from build123d import *

# Parameters (mm, degrees)
BOSS_EXTRUDE1_DEPTH     = 8
FILLET1_R               = 3
CUT_EXTRUDE1_DEPTH      = 90.03548582
CUT_EXTRUDE2_DEPTH      = 90.03548582
CUT_EXTRUDE2_DEPTH_BACK = 90.03548582
FILLET2_R               = 3
SKETCH4_R               = 1.5
CUT_EXTRUDE3_DEPTH      = 90.03548582
SKETCH5_R               = 2.5
CUT_EXTRUDE4_DEPTH      = 3
SKETCH7_W               = 100
SKETCH7_H               = 30
BOSS_EXTRUDE2_DEPTH     = 8
SKETCH8_W               = 15
SKETCH8_H               = 20
BOSS_EXTRUDE3_DEPTH     = 23
SKETCH9_R               = 2.5
CUT_EXTRUDE5_DEPTH      = 20
FILLET3_R               = 7.5
FILLET4_R               = 3
FILLET5_R               = 3
CUT_EXTRUDE6_DEPTH      = 142.723882577
CUT_EXTRUDE7_DEPTH      = 5
SKETCH12_W              = 15
SKETCH12_H              = 6
CUT_EXTRUDE8_DEPTH      = 5
SKETCH13_W              = 15
SKETCH13_H              = 6
CUT_EXTRUDE9_DEPTH      = 5
FILLET6_R               = 5


with BuildPart() as part:
    # Sketch1 → Boss-Extrude1 (new body)
    with BuildSketch(Plane(origin=(0, 0, 0), x_dir=(1, 0, 0), z_dir=(0, 1, 0))):
        Polygon((-10, 25), (0, 75), (10, 25), (25, 25), (25, 10), (75, 0), (25, -10), (25, -25), (10, -25), (0, -75), (-10, -25), (-25, -25), (-25, -10), (-75, 0), (-25, 10), (-25, 25), align=None)
    extrude(amount=BOSS_EXTRUDE1_DEPTH)

    # Fillet1
    fillet1_edges = [part.edges().sort_by_distance(p)[0] for p in [
        (0, 4, -75),
        (75, 4, 0),
        (0, 4, 75),
        (-75, 4, 0),
    ]]
    fillet(fillet1_edges, radius=FILLET1_R)

    # Sketch2 → Cut-Extrude1 (cut, symmetric)
    with BuildSketch(Plane(origin=(0, 0, 0), x_dir=(0, 0, -1), z_dir=(1, 0, 0))):
        Polygon((25, 8), (62.702941459, 2), (62.702941459, 8), align=None)
    cut_extrude1 = extrude(amount=CUT_EXTRUDE1_DEPTH, both=True, mode=Mode.SUBTRACT)

    # Mirror2: Cut-Extrude1 across plane
    add(cut_extrude1.mirror(Plane.XY), mode=Mode.SUBTRACT)

    # Sketch3 → Cut-Extrude2 (cut, two sides: drawn at the far end of the back side and taken through both)
    with BuildSketch(Plane.XY.offset(-CUT_EXTRUDE2_DEPTH_BACK)):
        Polygon((-25, 8), (-62.702941459, 2), (-62.702941459, 8), align=None)
    extrude(amount=CUT_EXTRUDE2_DEPTH + CUT_EXTRUDE2_DEPTH_BACK, mode=Mode.SUBTRACT)

    # Fillet2
    fillet2_edges = [part.edges().sort_by_distance(p)[0] for p in [
        (-10, 4, -25),
        (10, 4, -25),
        (25, 4, -25),
        (25, 4, 25),
        (10, 4, 25),
        (-10, 4, 25),
        (-25, 4, 25),
        (-25, 4, 10),
        (-25, 4, -10),
        (-25, 4, -25),
    ]]
    fillet(fillet2_edges, radius=FILLET2_R)

    # Sketch4 → Cut-Extrude3 (cut, through all)
    with BuildSketch(Plane(origin=(0, 8, 0), x_dir=(1, 0, 0), z_dir=(0, 1, 0))):
        with Locations(Location((-15.5, 15.5, 0), (0, 0, 270))):
            Circle(SKETCH4_R)
        with Locations(Location((15.5, 15.5, 0), (0, 0, 270))):
            Circle(SKETCH4_R)
        with Locations(Location((15.5, -15.5, 0), (0, 0, 270))):
            Circle(SKETCH4_R)
        with Locations(Location((-15.5, -15.5, 0), (0, 0, 270))):
            Circle(SKETCH4_R)
    extrude(amount=-CUT_EXTRUDE3_DEPTH, mode=Mode.SUBTRACT)

    # Sketch5 → Cut-Extrude4 (cut)
    with BuildSketch(Plane.XZ):
        with Locations(Location((15.5, -15.5, 0), (0, 0, 270))):
            Circle(SKETCH5_R)
        with Locations(Location((-15.5, -15.5, 0), (0, 0, 270))):
            Circle(SKETCH5_R)
        with Locations(Location((-15.5, 15.5, 0), (0, 0, 270))):
            Circle(SKETCH5_R)
        with Locations(Location((15.5, 15.5, 0), (0, 0, 270))):
            Circle(SKETCH5_R)
    extrude(amount=-CUT_EXTRUDE4_DEPTH, mode=Mode.SUBTRACT)

    # Sketch7 → Boss-Extrude2 (add)
    with BuildSketch(Plane(origin=(0, 8, 0), x_dir=(1, 0, 0), z_dir=(0, 1, 0))):
        with Locations((75, 0)):
            Rectangle(SKETCH7_W, SKETCH7_H)
    extrude(amount=-BOSS_EXTRUDE2_DEPTH)

    # Sketch8 → Boss-Extrude3 (add)
    with BuildSketch(Plane(origin=(0, 8, 0), x_dir=(1, 0, 0), z_dir=(0, 1, 0))):
        with Locations((117.5, 0)):
            Rectangle(SKETCH8_W, SKETCH8_H)
    extrude(amount=BOSS_EXTRUDE3_DEPTH)

    # Sketch9 → Cut-Extrude5 (cut)
    with BuildSketch(Plane.XY.offset(10)):
        with Locations((117.5, 25)):
            Circle(SKETCH9_R)
    extrude(amount=-CUT_EXTRUDE5_DEPTH, mode=Mode.SUBTRACT)

    # Fillet3
    fillet3_edges = [part.edges().sort_by_distance(p)[0] for p in [
        (110, 31, 0),
        (125, 31, 0),
    ]]
    fillet(fillet3_edges, radius=FILLET3_R - 0.0001)  # a hair under: the kernel refuses the full size

    # Fillet4
    fillet4_edges = [part.edges().sort_by_distance(p)[0] for p in [
        (117.5, 8, -10),
        (117.5, 8, 10),
    ]]
    fillet(fillet4_edges, radius=FILLET4_R)

    # Fillet5
    fillet5_edges = [part.edges().sort_by_distance(p)[0] for p in [
        (125, 4, 15),
        (125, 4, -15),
    ]]
    fillet(fillet5_edges, radius=FILLET5_R)

    # Sketch10 → Cut-Extrude6 (cut, through all)
    with BuildSketch(Plane(origin=(0, 8, 0), x_dir=(1, 0, 0), z_dir=(0, 1, 0))):
        Polygon((30, -8), (91.024338464, -8), (30, 5.94842022), align=None)
        Polygon((38.975661536, 8), (100, 8), (100, -5.94842022), align=None)
        Polygon((9.085786438, 10.5), (0, 1.414213562), (-9.085786438, 10.5), align=None)
        Polygon((10.5, -9.085786438), (1.414213562, 0), (10.5, 9.085786438), align=None)
        Polygon((-9.085786438, -10.5), (0, -1.414213562), (9.085786438, -10.5), align=None)
        Polygon((-10.5, 9.085786438), (-1.414213562, 0), (-10.5, -9.085786438), align=None)
    extrude(amount=-CUT_EXTRUDE6_DEPTH, mode=Mode.SUBTRACT)

    # Sketch11 → Cut-Extrude7 (cut)
    with BuildSketch(Plane.XY.offset(10)):
        with BuildLine():
            Line((109, 25), (109, 32))
            Line((109, 32), (126, 32))
            Line((126, 32), (126, 25))
            ThreePointArc((126, 25), (117.5, 16.5), (109, 25))
        make_face()
    cut_extrude7 = extrude(amount=-CUT_EXTRUDE7_DEPTH, mode=Mode.SUBTRACT)

    # Mirror4: Cut-Extrude7 across plane
    add(cut_extrude7.mirror(Plane.XY), mode=Mode.SUBTRACT)

    # Sketch12 → Cut-Extrude8 (cut)
    with BuildSketch(Plane.XY.offset(10)):
        with Locations((117.5, 18)):
            Rectangle(SKETCH12_W, SKETCH12_H)
    extrude(amount=-CUT_EXTRUDE8_DEPTH, mode=Mode.SUBTRACT)

    # Sketch13 → Cut-Extrude9 (cut)
    with BuildSketch(Plane(origin=(0, 0, -10), x_dir=(-1, 0, 0), z_dir=(0, 0, -1))):
        with Locations((-117.5, 18)):
            Rectangle(SKETCH13_W, SKETCH13_H)
    extrude(amount=-CUT_EXTRUDE9_DEPTH, mode=Mode.SUBTRACT)

    # Fillet6
    fillet6_edges = [part.edges().sort_by_distance(p)[0] for p in [
        (125, 15, -7.5),
        (110, 15, -7.5),
        (110, 15, 7.5),
        (125, 15, 7.5),
    ]]
    fillet(fillet6_edges, radius=FILLET6_R)


solid = part.part
Read the model definition and answer for the solid it produces. Units are mm, in the model's axes. A direction names the side the tool comes from. Round coordinates to 2 decimals unless told otherwise and drop trailing zeros. Write each loop counter-clockwise with the first axis right and the second up, starting at its lowest first coordinate (ties: lowest second). Pieces come first, ordered by that corner, then holes.
Q1. Find section A-A on x = 42. Determine the outline of the cut face in (y, z).
Values:
outline: (0, -15) - (8, -15) - (8, -8) - (0, -8) - close; (0, -7.31) - (8, -7.31) - (8, -3.21) - (0, -3.21) - close; (0, 8) - (8, 8) - (8, 15) - (0, 15) - close
Q2. A tool of negligible diameter and unlimited length cuts with its end or side. For faces 5 (the face through (0, 4, 10.5)), 6 (the face through (-17, 3, -17)), 7 (the face through (125, 9, 0)), from which of +Z, -Z, +X, -X, +Y, -Y can it reach the whole face along a straight path? Write none if from no direction.
Values:
face 5: +Y, -Y
face 6: -Y
face 7: +Z, -Z, +X, +Y, -Y
Q3. Straight lines are drawn through the part: line 1 (X direction, y = 6.8, z = 15.5); line 2 (X direction, y = 1.4, z = 15.5); line 3 (Z direction, x = 15, y = 1). For each, find the intervals that lie inside material, in ascending order.
Values:
line 1: x = -25 to -17, -14 to 14, 17 to 25
line 2: x = -25 to -18, -13 to 13, 18 to 25
line 3: z = -25 to -17.95, -13.05 to 13.05, 17.95 to 25
Q4. Flat-ended cylindrical pins translate along their axes: P1, Ø9, axis at x = 72, y = 2.5, coming from the +Z side; P2, Ø4, axis at x = 32.5, z = -12.5, coming from the -Y side; P3, Ø4, axis at x = 18.5, y = 5, coming from the +Z side; P4, Ø16.5, axis at x = 116.5, y = 17, coming from the -Z side. Find the tip coordinate at first contact, or state that the pin passes through.
Values:
P1: stops at z = 15
P2: stops at y = 0
P3: stops at z = 25
P4: stops at z = -11.02
Q5. Find section D-D on z = 44.5. Determine the outline of the cut face in (x, y).
Values:
outline: (-6.1, 0) - (6.1, 0) - (6.1, 4.9) - (-6.1, 4.9) - close
Q6. Find section C-C on z = -31. Determine the outline of the cut face in (x, y), and give its area (3 significant figures).
Values:
outline: (-8.8, 0) - (8.8, 0) - (8.8, 7.05) - (-8.8, 7.05) - close
area: 124 mm2
Q7. Find section B-B on x = 112. Determine the outline of the cut face in (y, z).
Values:
outline: (0, -15) - (8, -15) - (8, -13) arc R3 cw to (11, -10) - (14, -10) - (14, -5) - (28.6, -5) - (28.6, 5) - (14, 5) - (14, 10) - (11, 10) arc R3 cw to (8, 13) - (8, 15) - (0, 15) - close
Q8. The mould has two halves that part along X. Classify faces 1 (the face through (10.5, 4, 0)), 2 (the face through (-25, 4, 17)), 3 (the face through (-17, 1.5, -13.5)), 4 (the face through (117, 13, -10)): released by +X, released by -X, zero draft, split by the parting line, or undercut.
Values:
face 1: undercut
face 2: released by -X
face 3: undercut
face 4: zero draft
